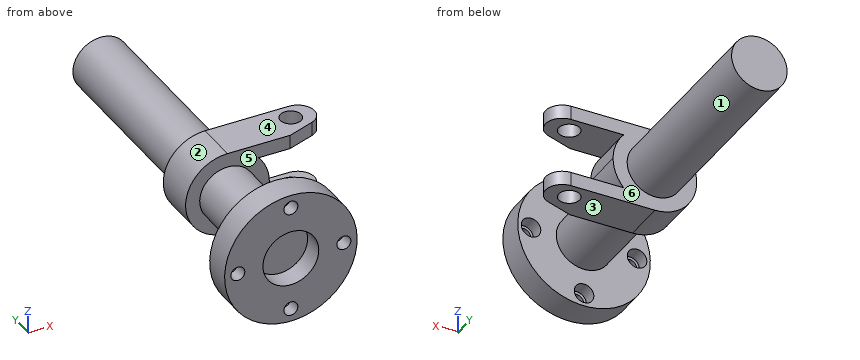
```python
from build123d import *

# Parameters (mm, degrees)
SKETCH3_R                                = 7.5
BOSS_EXTRUDE1_DEPTH                      = 47.5
BOSS_EXTRUDE1_DEPTH_BACK                 = 47.5
CUT_EXTRUDE1_REACH                       = 166.439
SKETCH4_W                                = 60
SKETCH4_H                                = 17.5
SKETCH4_W_2                              = 12
SKETCH4_H_2                              = 20
CBORE_FOR_M20_HEX_HEAD_BOLT1_D           = 10
CBORE_FOR_M20_HEX_HEAD_BOLT1_CBORE_D     = 14
CBORE_FOR_M20_HEX_HEAD_BOLT1_CBORE_DEPTH = 10


with BuildPart() as part:
    # Sketch2 → Revolve1 (revolve)
    with BuildSketch(Plane.XY, mode=Mode.PRIVATE) as revolve1_sk:
        Polygon((-47.5, 0), (-20, 0), (-20, 15), (0, 15), (0, 255), (-19.9, 255), (-19.9, 115), (-30, 115), (-30, 85), (-19.9, 85), (-19.9, 20), (-47.5, 20), align=None)
    revolve(revolve1_sk.sketch.rotate(Axis((0, 255, 0), (0, -1, 0)), 270), axis=Axis((0, 255, 0), (0, -1, 0)))

    # Sketch3 → Boss-Extrude1 (add, two sides)
    with BuildSketch(Plane.XY) as boss_extrude1_sk:
        with BuildLine():
            Line((0, 115), (60, 115))
            ThreePointArc((60, 115), (71.828663031, 105.020576871), (63.983453822, 91.680455148))
            Line((63.983453822, 91.680455148), (45, 85))
            Line((45, 85), (30, 85))
            Line((30, 85), (0, 85))
            Line((0, 85), (0, 115))
        make_face()
        with Locations((55, 103)):
            Circle(SKETCH3_R, mode=Mode.SUBTRACT)
    extrude(amount=BOSS_EXTRUDE1_DEPTH)
    extrude(boss_extrude1_sk.sketch, amount=-BOSS_EXTRUDE1_DEPTH_BACK)

    # Sketch4 → Cut-Extrude1 (cut, up to next)
    with BuildSketch(Plane(origin=(0, 115, 0), x_dir=(1, 0, 0), z_dir=(0, 1, 0)), mode=Mode.PRIVATE) as cut_extrude1_sk1:
        with Locations((30, -38.75)):
            Rectangle(SKETCH4_W, SKETCH4_H)
    cut_extrude1_tool1 = extrude(cut_extrude1_sk1.sketch, amount=-CUT_EXTRUDE1_REACH, mode=Mode.PRIVATE) & part.part
    # Sketch4 → Cut-Extrude1 (cut, up to next)
    with BuildSketch(Plane(origin=(0, 115, 0), x_dir=(1, 0, 0), z_dir=(0, 1, 0)), mode=Mode.PRIVATE) as cut_extrude1_sk2:
        with Locations((66, -38.75)):
            Rectangle(SKETCH4_W_2, SKETCH4_H)
    cut_extrude1_tool2 = extrude(cut_extrude1_sk2.sketch, amount=-CUT_EXTRUDE1_REACH, mode=Mode.PRIVATE) & part.part
    # Sketch4 → Cut-Extrude1 (cut, up to next)
    with BuildSketch(Plane(origin=(0, 115, 0), x_dir=(1, 0, 0), z_dir=(0, 1, 0)), mode=Mode.PRIVATE) as cut_extrude1_sk3:
        with BuildLine():
            ThreePointArc((30, 0), (28.025170769, -10.704662693), (22.360679775, -20))
            Line((22.360679775, -20), (60, -20))
            Line((60, -20), (60, 0))
            Line((60, 0), (30, 0))
        make_face()
    cut_extrude1_tool3 = extrude(cut_extrude1_sk3.sketch, amount=-CUT_EXTRUDE1_REACH, mode=Mode.PRIVATE) & part.part
    # Sketch4 → Cut-Extrude1 (cut, up to next)
    with BuildSketch(Plane(origin=(0, 115, 0), x_dir=(1, 0, 0), z_dir=(0, 1, 0)), mode=Mode.PRIVATE) as cut_extrude1_sk4:
        with Locations((66, -10)):
            Rectangle(SKETCH4_W_2, SKETCH4_H_2)
    cut_extrude1_tool4 = extrude(cut_extrude1_sk4.sketch, amount=-CUT_EXTRUDE1_REACH, mode=Mode.PRIVATE) & part.part
    # Sketch4 → Cut-Extrude1 (cut, up to next)
    with BuildSketch(Plane(origin=(0, 115, 0), x_dir=(1, 0, 0), z_dir=(0, 1, 0)), mode=Mode.PRIVATE) as cut_extrude1_sk5:
        with BuildLine():
            Line((60, 20), (22.360679775, 20))
            ThreePointArc((22.360679775, 20), (28.025170769, 10.704662693), (30, 0))
            Line((30, 0), (60, 0))
            Line((60, 0), (60, 20))
        make_face()
    cut_extrude1_tool5 = extrude(cut_extrude1_sk5.sketch, amount=-CUT_EXTRUDE1_REACH, mode=Mode.PRIVATE) & part.part
    # Sketch4 → Cut-Extrude1 (cut, up to next)
    with BuildSketch(Plane(origin=(0, 115, 0), x_dir=(1, 0, 0), z_dir=(0, 1, 0)), mode=Mode.PRIVATE) as cut_extrude1_sk6:
        with Locations((66, 10)):
            Rectangle(SKETCH4_W_2, SKETCH4_H_2)
    cut_extrude1_tool6 = extrude(cut_extrude1_sk6.sketch, amount=-CUT_EXTRUDE1_REACH, mode=Mode.PRIVATE) & part.part
    # Sketch4 → Cut-Extrude1 (cut, up to next)
    with BuildSketch(Plane(origin=(0, 115, 0), x_dir=(1, 0, 0), z_dir=(0, 1, 0)), mode=Mode.PRIVATE) as cut_extrude1_sk7:
        with Locations((30, 38.75)):
            Rectangle(SKETCH4_W, SKETCH4_H)
    cut_extrude1_tool7 = extrude(cut_extrude1_sk7.sketch, amount=-CUT_EXTRUDE1_REACH, mode=Mode.PRIVATE) & part.part
    # Sketch4 → Cut-Extrude1 (cut, up to next)
    with BuildSketch(Plane(origin=(0, 115, 0), x_dir=(1, 0, 0), z_dir=(0, 1, 0)), mode=Mode.PRIVATE) as cut_extrude1_sk8:
        with Locations((66, 38.75)):
            Rectangle(SKETCH4_W_2, SKETCH4_H)
    cut_extrude1_tool8 = extrude(cut_extrude1_sk8.sketch, amount=-CUT_EXTRUDE1_REACH, mode=Mode.PRIVATE) & part.part
    add(cut_extrude1_tool1.solids().sort_by_distance((30, 115, 38.75))[0], mode=Mode.SUBTRACT)
    add(cut_extrude1_tool2.solids().sort_by_distance((66, 115, 38.75))[0], mode=Mode.SUBTRACT)
    add(cut_extrude1_tool3.solids().sort_by_distance((43.723217, 115, 10.380581))[0], mode=Mode.SUBTRACT)
    add(cut_extrude1_tool4.solids().sort_by_distance((66, 115, 10))[0], mode=Mode.SUBTRACT)
    add(cut_extrude1_tool5.solids().sort_by_distance((43.723217, 115, -10.380581))[0], mode=Mode.SUBTRACT)
    add(cut_extrude1_tool6.solids().sort_by_distance((66, 115, -10))[0], mode=Mode.SUBTRACT)
    add(cut_extrude1_tool7.solids().sort_by_distance((30, 115, -38.75))[0], mode=Mode.SUBTRACT)
    add(cut_extrude1_tool8.solids().sort_by_distance((66, 115, -38.75))[0], mode=Mode.SUBTRACT)

    # CBORE for M20 Hex Head Bolt1 (through all)
    with Locations(Plane(origin=(0, 20, 0), x_dir=(1, 0, 0), z_dir=(0, 1, 0))):
        with Locations((38, 0), (0, 38), (-38, 0), (0, -38)):
            CounterBoreHole(CBORE_FOR_M20_HEX_HEAD_BOLT1_D / 2, CBORE_FOR_M20_HEX_HEAD_BOLT1_CBORE_D / 2, CBORE_FOR_M20_HEX_HEAD_BOLT1_CBORE_DEPTH)


solid = part.part
```
The model under review builds one solid part; all positions refer to its coordinate system, in mm. Face numbers are marked on the shaded views. A direction names the side the tool comes from. Coordinates: 2 decimals unless noted, no trailing zeros. Write each loop counter-clockwise with the first axis right and the second up, starting at its lowest first coordinate (ties: lowest second). Pieces come first, ordered by that corner, then holes. Notation, with made-up numbers: (-25.75, 61.25) -> (-10.75, 61.25) arc R14 ccw to (-10.75, 87.25) -> close; hole circle Ø11 at (29.25, -20.75). An arc over 180 degrees is marked (long way). One line per item, written item: value. Start each with the question number.
Q1. Add section B-B, the plane x = 38. Give the boundary of the cut face in (y, z).
Q2. Add section A-A, the plane z = -38. Give the boundary of the cut face in (x, y).
Q3. To check wall thickness, follow probe 1 along Y at (x, z) = (25, 14.5); probe 2 along Y at (x, z) = (9.5, -12); probe 3 along Y at (x, z) = (-29.5, 22). State the ranges of each line that lie inside material, in increasing order.
Q4. Clearance check with flat-ended pins moving along their axes: P1, Ø24, axis at x = 23.5, y = 106, coming from the -Z side; P2, Ø12, axis at x = -0.5, z = 2.5, coming from the -Y side; P3, Ø6, axis at x = -26.5, z = -17, coming from the +Y side. State where each tip first meets the part, or that it passes through.
Q5. Add section C-C, the plane y = 103. Give the boundary of the cut face in (x, z), then the cut area to 3 significant figures.
Q6. The part is to be moulded in two halves that separate along Y. For the marked faces 4, 5 and 6, say which applies: +Y half, -Y half, draft (parallel to the pull), parting line (faces both ways), or undercut.
Q7. For the marked faces 1, 2 and 3, list the 3-axis set-ups (+Z, -Z, +X, -X, +Y, -Y) from which the entire face can be reached by the end or side of a thin tool; tool diameter is ignored.
Q8. Add section D-D, the plane z = 22.5. Give the boundary of the cut face in (x, y).
Response:
1. outline: (0, -28.5) -> (20, -28.5) -> (20, -7) -> (10, -7) -> (10, -5) -> (0, -5) -> close; (0, 5) -> (10, 5) -> (10, 7) -> (20, 7) -> (20, 28.5) -> (0, 28.5) -> close; (85, -30) -> (115, -30) -> (115, -20) -> (85, -20) -> close; (85, 20) -> (115, 20) -> (115, 30) -> (85, 30) -> close
2. outline: (-28.5, 0) -> (-5, 0) -> (-5, 10) -> (-7, 10) -> (-7, 20) -> (-28.5, 20) -> close; (5, 0) -> (28.5, 0) -> (28.5, 20) -> (7, 20) -> (7, 10) -> (5, 10) -> close
3. probe 1: 0 to 20, 85 to 115
3. probe 2: 15 to 255
3. probe 3: 0 to 20
4. P1: z = -30
4. P2: y = 15
4. P3: y = 115
5. outline: (0, -30) -> (47.5, -30) -> (47.5, -20) -> (22.36, -20) arc R30 ccw to (22.36, 20) -> (47.5, 20) -> (47.5, 30) -> (0, 30) arc R30 ccw to start; (62.5, -30) -> (72, -30) -> (72, -20) -> (62.5, -20) -> close; (62.5, 20) -> (72, 20) -> (72, 30) -> (62.5, 30) -> close
5. area: 3,660 mm²
6. face 4: draft
6. face 5: undercut
6. face 6: +Y half
7. face 1: +Y
7. face 2: -X, +Y
7. face 3: -Z, +X, -X, +Y
8. outline: (-41.83, 0) -> (41.83, 0) -> (41.83, 20) -> (-41.83, 20) -> close; (-19.84, 85) -> (45, 85) -> (63.98, 91.68) arc R12 ccw to (60, 115) -> (-19.84, 115) -> close; hole circle Ø15 at (55, 103)
